from build123d import *

# Parameters (mm, degrees)
F0_W      = 130
F0_H      = 42
F0_W_2    = 90
F0_H_2    = 36
F1_DEPTH  = 4
F3_DEPTH  = 5
F5_DEPTH  = 3
F6_SIZE   = 3
F7_R      = 3
F8_DEPTH  = 12.5
F10_R     = 3
F11_DEPTH = 37.9
F12_W     = 130
F12_H     = 42
F13_DEPTH = 20
F14_W     = 3.5
F14_H     = 10.9
F15_DEPTH = 8


with BuildPart() as f1:
    # F0 (on Top) → F1 (new body)
    with BuildSketch(Plane.XY):
        Rectangle(F0_W, F0_H)
        Rectangle(F0_W_2, F0_H_2, mode=Mode.SUBTRACT)
    extrude(amount=F1_DEPTH)

    # F2 (on face) → F3 (join)
    with BuildSketch(Plane.XY.offset(4)):
        Polygon((45, 7.1), (45, 4.1), (56, 4.1), (60.1, 0), (56, -4.1), (45, -4.1), (45, -7.1), (57.242641, -7.1), (64.342641, 0), (57.242641, 7.1), align=None)
    extrude(amount=F3_DEPTH)

    # F4 (on face) → F5 (join)
    with BuildSketch(Plane.XY.offset(9)):
        Polygon((57.242641, 7.1), (45, 7.1), (45, -7.1), (57.242641, -7.1), (64.342641, 0), align=None)
        Polygon((57.242641, 7.1), (45, 7.1), (45, -4.1), (45, -7.1), (57.242641, -7.1), (64.342641, 0), align=None)
    extrude(amount=F5_DEPTH)

    # F6
    f6_edges = [f1.edges().sort_by_distance(p)[0] for p in [
        (64.342641, 0, 8),
    ]]
    chamfer(f6_edges, length=F6_SIZE)

    # F7 (on face) → F8 (cut, symmetric)
    with BuildSketch(Plane.XY.offset(4)):
        with Locations((55.5, 0.032705)):
            Circle(F7_R)
    extrude(amount=F8_DEPTH, both=True, mode=Mode.SUBTRACT)

    # F9: F1 across plane


with BuildPart() as f1_1:
    add(f1.part)
    add(f1.part.mirror(Plane.YZ))

    # F10 (on face) → F11 (cut)
    with BuildSketch(Plane.XY.offset(12)):
        with Locations((-55.5, 0.032705)):
            Circle(F10_R)
        with Locations((55.5, 0.032705)):
            Circle(F10_R)
    extrude(amount=-F11_DEPTH, mode=Mode.SUBTRACT)

    # F12 (on face) → F13 (join)
    with BuildSketch(Plane.XY.offset(4)):
        Rectangle(F12_W, F12_H)
        Polygon((45, 18), (62.22132, 18), (62.22132, 2.12132), (62.22132, -2.12132), (62.22132, -18), (45, -18), (-45, -18), (-62.22132, -18), (-62.22132, -2.12132), (-62.22132, 2.12132), (-62.22132, 18), (-45, 18), align=None, mode=Mode.SUBTRACT)
    extrude(amount=F13_DEPTH)

    # F14 (on face) → F15 (join)
    with BuildSketch(Plane.XY.offset(4)):
        with Locations((-46.75, 12.55)):
            Rectangle(F14_W, F14_H)
    extrude(amount=F15_DEPTH)

    # F16: F1 across plane


with BuildPart() as f1_2:
    add(f1_1.part)
    add(f1_1.part.mirror(Plane.XZ))

    # F17: F1 across plane


with BuildPart() as f1_3:
    add(f1_2.part)
    add(f1_2.part.mirror(Plane.YZ))


solid = f1_3.part
Verification items for the finished model (mm, model axes). A direction names the side the tool comes from. Coordinates: 2 decimals unless noted, no trailing zeros. Loops run counter-clockwise (first coordinate to the right, second up) from the corner with the lowest first, then second, coordinate; pieces in that order, holes last. Notation, with made-up numbers: (-37.75, 86.25) -> (-11.75, 86.25) arc R15 cw to (-11.75, 98.25) -> close; hole circle Ø3 at (-26.75, 60). An arc over 180 degrees is marked (long way). Answer as CSV lines item,"result".
1) Cross-section at B-B, the plane z = 16.25. Record the cut outline in (x, y).
Found:
outline,"(-65, -21) -> (65, -21) -> (65, 21) -> (-65, 21) -> close; hole (-62.22, -18) -> (62.22, -18) -> (62.22, 18) -> (-62.22, 18) -> close"
2) Cross-section at C-C, the plane x = -6. Record the cut outline in (y, z), then the cut area to 3 significant figures.
Found:
outline,"(-21, 0) -> (-18, 0) -> (-18, 24) -> (-21, 24) -> close; (18, 0) -> (21, 0) -> (21, 24) -> (18, 24) -> close"
area,"144 mm2"
3) Depth check by flat-ended pin: pin 1 (4 mm diameter, centred on x = -52, y = -1, fed in from +Z). Enter the tip coordinate at first touch or a pass-through.
Found:
pin 1,"stops at z = 12"
4) Cross-section at D-D, the plane z = 5.75. Count the separate pieces of the cut face and the enclosed holes in it, then the cut area to 3 significant figures.
Found:
separate pieces,"1"
enclosed holes,"5"
area,"1,360 mm2"
5) Thickness scan on L1, parallel to X at y = -10, z = 7.5; L2, parallel to Y at x = 18.5, z = 12; L3, parallel to X at y = -8.5, z = 19. Record the ranges inside material, lowest first. Write a range as from..to.
Found:
L1,"x = -65..-62.22, -48.5..-45, 45..48.5, 62.22..65"
L2,"y = -21..-18, 18..21"
L3,"x = -65..-62.22, 62.22..65"
6) Cross-section at A-A, the plane y = 16. Record the cut outline in (x, z), then the cut area to 3 significant figures.
Found:
outline,"(-65, 0) -> (-45, 0) -> (-45, 12) -> (-48.5, 12) -> (-48.5, 4) -> (-62.22, 4) -> (-62.22, 24) -> (-65, 24) -> close; (45, 0) -> (65, 0) -> (65, 24) -> (62.22, 24) -> (62.22, 4) -> (48.5, 4) -> (48.5, 12) -> (45, 12) -> close"
area,"327 mm2"
7) Tool access check on faces 4 (the flat face through (53, -7.1, 8)), 5 (the flat face through (-45, 0, 3)), 6 (the flat face through (51, 0, 9)). Record the directions out of +Z, -Z, +X, -X, +Y, -Y that give a thin tool (end or side, any length) a straight path to the whole face; none if there is none.
Found:
face 4,"+Z"
face 5,"+Z, -Z"
face 6,"none"
8) Release check for a two-part mould opening along X. For faces 1 (the flat face through (65, 0, 12)), 2 (the flat face through (58, 2.1, 6.5)), 3 (the flat face through (48.5, -12, 8)) record: +X half, -X half, draft (parallel to the pull), parting line (faces both ways), or undercut.
Found:
face 1,"+X half"
face 2,"undercut"
face 3,"undercut"
